from build123d import *

# Parameters (mm, degrees)
F0_W            = 76.2
F0_H            = 76.2
F1_DEPTH        = 35.56
F0_W_2          = 71.12
F2_DEPTH        = 71.12
F4_DEPTH        = 76.201
F5_R            = 10.16
F6_DEPTH        = 76.201
F8_DEPTH        = 71.121
F10_D           = 15.24
F10_CBORE_D     = 40.64
F10_CBORE_DEPTH = 10.16
F11_W           = 10.16
F11_H           = 10.16
F12_DEPTH       = 76.2
F13_R           = 10.16


with BuildPart() as f1:
    # F0 (on Top) → F1 (new body)
    with BuildSketch(Plane.XY):
        with Locations((38.1, 38.1)):
            Rectangle(F0_W, F0_H)
    extrude(amount=F1_DEPTH)

    # F0 (on Top) → F2 (join)
    with BuildSketch(Plane.XY):
        with Locations((111.76, 38.1)):
            Rectangle(F0_W_2, F0_H)
    extrude(amount=F2_DEPTH)

    # F3 (on face) → F4 (cut, through all)
    with BuildSketch(Plane.XZ):
        Polygon((76.2, 35.56), (111.76, 71.12), (76.2, 71.12), align=None)
        Polygon((111.76, 0), (147.32, 0), (147.32, 35.56), align=None)
    extrude(amount=-F4_DEPTH, mode=Mode.SUBTRACT)

    # F5 (on face) → F6 (cut, through all)
    with BuildSketch(Plane.XZ):
        with Locations((93.98, 20.32)):
            Circle(F5_R)
    extrude(amount=-F6_DEPTH, mode=Mode.SUBTRACT)

    # F7 (on face) → F8 (cut, through all)
    with BuildSketch(Plane.XY.offset(71.12)):
        with BuildLine():
            ThreePointArc((137.16, 60.96), (129.54, 68.58), (121.92, 60.96))
            Line((121.92, 60.96), (121.92, 15.24))
            ThreePointArc((121.92, 15.24), (129.54, 7.62), (137.16, 15.24))
            Line((137.16, 15.24), (137.16, 60.96))
        make_face()
    extrude(amount=-F8_DEPTH, mode=Mode.SUBTRACT)

    # F10 (through all)
    with Locations(Plane.XY.offset(35.56)):
        with Locations((38.1, 38.1)):
            CounterBoreHole(F10_D / 2, F10_CBORE_D / 2, F10_CBORE_DEPTH)

    # F11 (on face) → F12 (cut)
    with BuildSketch(Plane(origin=(0, 0, 0), x_dir=(0, -1, 0), z_dir=(-1, 0, 0))):
        with Locations((-38.1, 30.48)):
            Rectangle(F11_W, F11_H)
    extrude(amount=-F12_DEPTH, mode=Mode.SUBTRACT)

    # F13
    f13_edges = [f1.edges().sort_by_distance(p)[0] for p in [
        (0, 76.2, 17.78),
        (0, 0, 17.78),
    ]]
    fillet(f13_edges, radius=F13_R)


solid = f1.part
Read the model definition and answer for the solid it produces. Units are mm, in the model's axes. A direction names the side the tool comes from. Give positions to 0.01 mm unless a question says otherwise; leave off trailing zeros. Write each loop counter-clockwise with the first axis right and the second up, starting at its lowest first coordinate (ties: lowest second). Pieces come first, ordered by that corner, then holes. Notation, with made-up numbers: (39.5, 4.5) -> (70.5, 4.5) arc R31 cw to (70.5, 31.5) -> close; hole circle Ø2 at (64, -30.5). An arc over 180 degrees is marked (long way). Answer as a JSON object with one key per item and string values. Group by question number.
1) Find section B-B (x = 129.54). Write down the section's boundary in (y, z), and give its area (3 significant figures).
2) Find section A-A (y = 38.1). Write down the section's boundary in (x, z).
3) Find section D-D (y = 26). Write down the section's boundary in (x, z).
4) Each of these flat-tipped pins is pushed along its axis until it touches: P1, Ø5, axis at y = 36, z = 30.5, coming from the -X side; P2, Ø20.5, axis at x = 21, y = 30.5, coming from the +Z side; P3, Ø3, axis at x = 131.5, y = 66, coming from the +Z side; P4, Ø17.5, axis at x = 38.1, y = 38.1, coming from the +Z side. Where does it stop, or does it pass through?
5) A tool of negligible diameter and unlimited length cuts with its end or side. For faces 4 (the flat face through (46, 38, 25.4)), 5 (the flat face through (9, 33.02, 30)), 6 (the flat face through (137.16, 38, 49)), from which of +Z, -Z, +X, -X, +Y, -Y can it reach the whole face along a straight path? Write none if from no direction.
6) Consider L1, parallel to Y at x = 38.1, z = 7; L2, parallel to X at y = 29, z = 27; L3, parallel to X at y = 49.5, z = 34.5. Determine where each line is inside the solid, lowest interval first. Write a range as from..to.
7) The mould has two halves that part along X. Classify faces 1 (the flat face through (76.2, 38, 31)), 2 (the flat face through (121.92, 38, 41)), 3 (the flat face through (38, 13, 35.56)): +X half, -X half, draft (parallel to the pull), parting line (faces both ways), or undercut.
8) Find section C-C (z = 20.32). Write down the section's boundary in (x, y).
Values follow:
{
 "1": {"outline": "(0, 17.78) -> (7.62, 17.78) -> (7.62, 71.12) -> (0, 71.12) -> close; (68.58, 17.78) -> (76.2, 17.78) -> (76.2, 71.12) -> (68.58, 71.12) -> close", "area": "813 mm2"},
 "2": {"outline": "(0, 0) -> (30.48, 0) -> (30.48, 25.4) -> (0, 25.4) -> close; (45.72, 0) -> (111.76, 0) -> (121.92, 10.16) -> (121.92, 71.12) -> (111.76, 71.12) -> (76.2, 35.56) -> (76.2, 25.4) -> (45.72, 25.4) -> close; (137.16, 25.4) -> (147.32, 35.56) -> (147.32, 71.12) -> (137.16, 71.12) -> close; hole circle Ø20.32 at (93.98, 20.32)"},
 "3": {"outline": "(0, 0) -> (111.76, 0) -> (121.92, 10.16) -> (121.92, 71.12) -> (111.76, 71.12) -> (76.2, 35.56) -> (54.42, 35.56) -> (54.42, 25.4) -> (21.78, 25.4) -> (21.78, 35.56) -> (0, 35.56) -> close; (137.16, 25.4) -> (147.32, 35.56) -> (147.32, 71.12) -> (137.16, 71.12) -> close; hole circle Ø20.32 at (93.98, 20.32)"},
 "4": {"P1": "stops at x = 76.2", "P2": "stops at z = 35.56", "P3": "passes through", "P4": "stops at z = 25.4"},
 "5": {"face 4": "+Z", "face 5": "+Z, -X", "face 6": "+Z, -Z"},
 "6": {"L1": "y = 0..30.48, 45.72..76.2", "L2": "x = 0..19.93, 56.27..86.32, 101.64..121.92, 137.16..138.76", "L3": "x = 0..21.28, 54.92..121.92, 137.16..146.26"},
 "7": {"face 1": "-X half", "face 2": "undercut", "face 3": "draft"},
 "8": {"outline": "(0, 10.16) arc R10.16 ccw to (10.16, 0) -> (83.82, 0) -> (83.82, 76.2) -> (10.16, 76.2) arc R10.16 ccw to (0, 66.04) -> close; (104.14, 0) -> (132.08, 0) -> (132.08, 8.06) arc R7.62 cw to (121.92, 15.24) -> (121.92, 60.96) arc R7.62 cw to (132.08, 68.14) -> (132.08, 76.2) -> (104.14, 76.2) -> close; hole circle Ø15.24 at (38.1, 38.1)"}
}
